from build123d import *

# Parameters (mm, degrees)
CROQUIS1_R                 = 1.6
SALIENTE_EXTRUIR1_DEPTH    = 10
CORTAR_EXTRUIR1_DEPTH      = 8.1
CORTAR_EXTRUIR1_DEPTH_BACK = 8.1
CORTAR_EXTRUIR2_START      = 8.1
CROQUIS3_OUTSIDE_W         = 34.658
CROQUIS3_OUTSIDE_H         = 30.658
CROQUIS3_OUTSIDE_W_2       = 10
CROQUIS3_OUTSIDE_H_2       = 25.797501395
CORTAR_EXTRUIR2_DEPTH      = 8
CROQUIS4_W                 = 10
CROQUIS4_H                 = 8
SALIENTE_EXTRUIR3_DEPTH    = 3
CORTAR_EXTRUIR3_DEPTH      = 25.088378941
CORTAR_EXTRUIR3_DEPTH_BACK = 25.088378941
CROQUIS5_W                 = 8.1
CROQUIS5_H                 = 3.5
CROQUIS6_R                 = 4.5
CROQUIS6_R_2               = 1.6
SALIENTE_EXTRUIR4_DEPTH    = 3
CHAFL_N1_SIZE              = 1
CROQUIS7_R                 = 3.5
CORTAR_EXTRUIR4_DEPTH      = 3
CHAFL_N2_SIZE              = 1


with BuildPart() as part:
    # Croquis1 → Saliente-Extruir1 (new, symmetric)
    with BuildSketch(Plane.XY):
        with BuildLine():
            Line((-12.5, -15), (-5.566639674, 2.238866395))
            ThreePointArc((-5.566639674, 2.238866395), (0, 6), (5.566639674, 2.238866395))
            Line((5.566639674, 2.238866395), (12.5, -15))
            Line((12.5, -15), (-12.5, -15))
        make_face()
        Circle(CROQUIS1_R, mode=Mode.SUBTRACT)
    extrude(amount=SALIENTE_EXTRUIR1_DEPTH, both=True)

    # Croquis2 → Cortar-Extruir1 (cut, two sides: drawn at the far end of the back side and taken through both)
    with BuildSketch(Plane.XY.offset(-CORTAR_EXTRUIR1_DEPTH_BACK)):
        with BuildLine():
            Line((-12.5, -15), (-7.5, 0))
            ThreePointArc((-7.5, 0), (0, 7.5), (7.5, 0))
            Line((7.5, 0), (12.5, -15))
            Line((12.5, -15), (2.888582809, -8))
            Line((2.888582809, -8), (-3.164835235, -8))
            Line((-3.164835235, -8), (-12.5, -15))
        make_face()
    extrude(amount=CORTAR_EXTRUIR1_DEPTH + CORTAR_EXTRUIR1_DEPTH_BACK, mode=Mode.SUBTRACT)

    # Croquis3 outside → Cortar-Extruir2 (cut)
    with BuildSketch(Plane.XY.offset(CORTAR_EXTRUIR2_START)):
        with Locations((0, -4.5)):
            Rectangle(CROQUIS3_OUTSIDE_W, CROQUIS3_OUTSIDE_H)
        with Locations((0, -2.101249303)):
            Rectangle(CROQUIS3_OUTSIDE_W_2, CROQUIS3_OUTSIDE_H_2, mode=Mode.SUBTRACT)
    extrude(amount=-CORTAR_EXTRUIR2_DEPTH, mode=Mode.SUBTRACT)

    # Croquis4 → Saliente-Extruir3 (add)
    with BuildSketch(Plane.XZ.offset(15)):
        with Locations((0, 4.1)):
            Rectangle(CROQUIS4_W, CROQUIS4_H)
    extrude(amount=SALIENTE_EXTRUIR3_DEPTH)

    # Croquis5 → Cortar-Extruir3 (cut, two sides: drawn at the far end of the back side and taken through both)
    with BuildSketch(Plane(origin=(0, 0, 0), x_dir=(0, 0, -1), z_dir=(1, 0, 0)).offset(-CORTAR_EXTRUIR3_DEPTH_BACK)):
        with Locations((4.05, -9.75)):
            Rectangle(CROQUIS5_W, CROQUIS5_H)
    extrude(amount=CORTAR_EXTRUIR3_DEPTH + CORTAR_EXTRUIR3_DEPTH_BACK, mode=Mode.SUBTRACT)

    # Croquis6 → Saliente-Extruir4 (add)
    with BuildSketch(Plane.XY.offset(-8.1)):
        Circle(CROQUIS6_R)
        Circle(CROQUIS6_R_2, mode=Mode.SUBTRACT)
    extrude(amount=SALIENTE_EXTRUIR4_DEPTH)

    # Chaflán1
    chafl_n1_edges = [part.edges().sort_by_distance(p)[0] for p in [
        (-4.5, 0, -5.1),
    ]]
    chamfer(chafl_n1_edges, length=CHAFL_N1_SIZE)

    # Croquis7 → Cortar-Extruir4 (cut)
    with BuildSketch(Plane(origin=(0, 0, -10), x_dir=(-1, 0, 0), z_dir=(0, 0, -1))):
        Circle(CROQUIS7_R)
    extrude(amount=-CORTAR_EXTRUIR4_DEPTH, mode=Mode.SUBTRACT)

    # Chaflán2
    chafl_n2_edges = [part.edges().sort_by_distance(p)[0] for p in [
        (-9.033319837, -6.380566802, -10),
        (0, 6, -10),
        (9.033319837, -6.380566802, -10),
    ]]
    chamfer(chafl_n2_edges, length=CHAFL_N2_SIZE)


solid = part.part
Verification items for the finished model (mm, model axes). A direction names the side the tool comes from. Round coordinates to 2 decimals unless told otherwise and drop trailing zeros. Loops run counter-clockwise (first coordinate to the right, second up) from the corner with the lowest first, then second, coordinate; pieces in that order, holes last. Notation, with made-up numbers: (34, 45) - (85, 45) arc R14 cw to (85, 65) - close; hole circle Ø8 at (69.25, -2). An arc over 180 degrees is marked (long way). Use a Markdown table: item, result. Add a question column.
1. Section check C-C, the plane y = -7. Record the boundary of the cut face in (x, z), plus the area to 3 significant figures.
2. Section check D-D, the plane x = -6.75. Record the boundary of the cut face in (y, z).
3. Section check B-B, the plane z = -7.5. Record the boundary of the cut face in (x, y).
4. Release check for a two-part mould opening along Y. For faces 1 (the face through (-1, -2, -7)), 2 (the face through (1, -2, -5.1)), 3 (the face through (8.83, -12.327, -1.913)) record: released by +Y, released by -Y, zero draft, split by the parting line, or undercut.
5. Thickness scan on probe 1 along Z at (x, y) = (0.5, -6.75); probe 2 along Y at (x, z) = (0, -8.85); probe 3 along Z at (x, y) = (-0.25, 2). Record the ranges inside material, lowest first. Write a range as [from, to].
6. Gauge pin test, flat ends, axial feed: pin 1 (3 mm diameter, centred on x = -1.5, z = 2, fed in from +Y); pin 2 (5.5 mm diameter, centred on x = 0, y = 0, fed in from +Z); pin 3 (8 mm diameter, centred on x = -6, z = -4, fed in from -Y); pin 4 (3.5 mm diameter, centred on x = 1.5, y = -0.5, fed in from -Z). Record the tip position at first contact, or that the pin passes through.
7. Section check A-A, the plane x = 0. Give the number of separate pieces and of enclosed holes in the cut face, plus the area to 3 significant figures.
8. Access from +Z, -Z, +X, -X, +Y, -Y to the whole of each face (thin tool, end or side, straight path). Record for faces 4 (the face through (0, -16, 8.1)), 5 (the face through (0, -15, -5)), 6 (the face through (0, -4, 8.1)), 7 (the face through (0, -10, 0)), 8 (the face through (0, -7, -8.1)).
Checks:
| question | item | result |
|---|---|---|
| 1 | outline | (-9.28, -9) - (-8.2, -10) - (8.2, -10) - (9.28, -9) - (9.28, -8.1) - (-9.28, -8.1) - close; (-9.28, 8.1) - (9.28, 8.1) - (9.28, 10) - (-9.28, 10) - close |
| 1 | area | 69.5 mm^2 |
| 2 | outline | (-15, -10) - (-3.38, -10) - (-0.7, -9) - (-0.7, -8.1) - (-11.5, -8.1) - (-11.5, 0) - (-10.69, 0) - (-10.69, 0.1) - (-15, 0.1) - close; (-15, 8.1) - (-0.7, 8.1) - (-0.7, 10) - (-15, 10) - close |
| 3 | outline | (-12.5, -15) - (12.5, -15) - (7.69, -11.5) - (-7.83, -11.5) - close; circle Ø9 at (0, 0); hole circle Ø7 at (0, 0) |
| 4 | face 1 | undercut |
| 4 | face 2 | zero draft |
| 4 | face 3 | released by +Y |
| 5 | probe 1 | z = [-10, -8.1], [8.1, 10] |
| 5 | probe 2 | y = [-15, -3.5], [3.5, 6] |
| 5 | probe 3 | z = [-7, -5.1], [8.1, 10] |
| 6 | pin 1 | stops at y = -8 |
| 6 | pin 2 | stops at z = 10 |
| 6 | pin 3 | stops at y = -15 |
| 6 | pin 4 | stops at z = -7 |
| 7 | separate pieces | 3 |
| 7 | enclosed holes | 0 |
| 7 | area | 181 mm^2 |
| 8 | face 4 | +Z, +X, -X, -Y |
| 8 | face 5 | -Z, +X, -X, -Y |
| 8 | face 6 | +Y |
| 8 | face 7 | +X, -X, +Y |
| 8 | face 8 | none |
